```python
from build123d import *

# Parameters (mm, degrees)
F1_DEPTH = 5


# Not quite as in the source:
# - a feature of the source that left no trace in its solid (it failed there, or was rolled back) is left out


with BuildPart() as f1:
    # F0 (on Front) → F1 (new body)
    with BuildSketch(Plane.XZ):
        Polygon((32.530919835, 39.797769749), (-17.469080165, 39.797769749), (-17.469080165, 33.1753157079), (-7.3289242573, 33.1753157079), (22.6710757427, 33.1753157079), (32.530919835, 33.1753157079), align=None)
        with BuildLine():
            Line((22.6710757427, 33.1753157079), (-7.3289242573, 33.1753157079))
            ThreePointArc((-7.3289242573, 33.1753157079), (-3.5071800034, 30.8135939836), (0.6755496306, 29.1740112764))
            Line((0.6755496306, 29.1740112764), (7.6710757427, 29.1740112764))
            Line((7.6710757427, 29.1740112764), (14.6666018548, 29.1740112764))
            ThreePointArc((14.6666018548, 29.1740112764), (18.8493314888, 30.8135939836), (22.6710757427, 33.1753157079))
        make_face()
        with BuildLine():
            Line((7.6710757427, 29.1740112764), (0.6755496306, 29.1740112764))
            ThreePointArc((0.6755496306, 29.1740112764), (0.5215760436, 24.0947560366), (5.6017371537, 24.215191712))
            ThreePointArc((5.6017371537, 24.215191712), (6.355285365, 26.8119146366), (7.6710757427, 29.1740112764))
        make_face()
        with BuildLine():
            ThreePointArc((9.7404143316, 24.215191712), (15.0089010531, 23.907669722), (14.6666018548, 29.1740112764))
            Line((14.6666018548, 29.1740112764), (7.6710757427, 29.1740112764))
            ThreePointArc((7.6710757427, 29.1740112764), (8.9868661204, 26.8119146366), (9.7404143316, 24.215191712))
        make_face()
        with BuildLine():
            ThreePointArc((9.7404143316, 24.215191712), (8.9868661204, 26.8119146366), (7.6710757427, 29.1740112764))
            ThreePointArc((7.6710757427, 29.1740112764), (6.355285365, 26.8119146366), (5.6017371537, 24.215191712))
            ThreePointArc((5.6017371537, 24.215191712), (5.7343151874, 19.5038742549), (7.6710757427, 15.20700939))
            ThreePointArc((7.6710757427, 15.20700939), (9.607836298, 19.5038742549), (9.7404143316, 24.215191712))
        make_face()
    extrude(amount=F1_DEPTH)


solid = f1.part
```
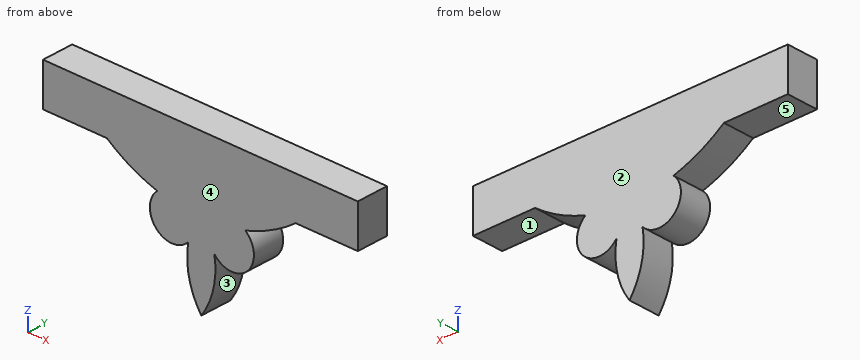
Model file for the job. Use its own axes, mm. Face numbers are marked on the shaded views. A direction names the side the tool comes from. Coordinates: 2 decimals unless noted, no trailing zeros. Order: outer loops, then holes, each group sorted by start corner. A loop starts at its lowest first (then second) coordinate and runs counter-clockwise, first axis right, second up. Notation, with made-up numbers: (-9, 52.5) - (33, 52.5) arc R24 ccw to (33, 81.5) - close; hole circle Ø5 at (-32.75, -15.5). An arc over 180 degrees is marked (long way). Return JSON: item names as keys, results as strings. Group by question number.
1) Saw through at A-A, the plane y = -1.3. Write the cut outline in (x, z).
2) Saw through at B-B, the plane x = 15.5. Write the cut outline in (y, z).
3) Probe line 1 (X direction, y = -4.4, z = 23.5); line 2 (Z direction, x = -10, y = -3.4); line 3 (X direction, y = -4.55, z = 24.75). List the from-to ranges inside material, lowest first. Write a range as from..to.
4) Saw through at D-D, the plane z = 31.5. Write the cut outline in (x, y), plus the area to 3 significant figures.
5) Tool access for the marked faces 1 and 2: list every direction of +Z, -Z, +X, -X, +Y, -Y with a clear straight run to the whole face (end or side of a thin tool).
6) Saw through at C-C, the plane x = 27.5. Write the cut outline in (y, z).
7) Flat gauge pins, fed straight in: P1, Ø2.5, axis at x = -15, y = -3, coming from the -Z side; P2, Ø3, axis at x = 15.5, y = -1, coming from the -Z side; P3, Ø1, axis at x = 20.5, y = -4, coming from the -Z side. Where does each tip first touch, or does it go through?
8) Mould opens along Z. For the marked faces 3, 4 and 5 say: released by +Z, released by -Z, zero draft, split by the parting line, or undercut.
Values found:
{
 "1": {"outline": "(-17.47, 33.18) - (-7.33, 33.18) arc R25 ccw to (0.68, 29.17) arc R3.5 ccw (long way) to (5.6, 24.22) arc R12 ccw to (7.67, 15.21) arc R12 ccw to (9.74, 24.22) arc R3.52 ccw (long way) to (14.67, 29.17) arc R25 ccw to (22.67, 33.18) - (32.53, 33.18) - (32.53, 39.8) - (-17.47, 39.8) - close"},
 "2": {"outline": "(-5, 24.53) - (0, 24.53) - (0, 28.25) - (-5, 28.25) - close; (-5, 29.43) - (0, 29.43) - (0, 39.8) - (-5, 39.8) - close"},
 "3": {"line 1": "x = 1.31..4.7, 5.5..9.84, 10.5..14.52", "line 2": "z = 33.18..39.8", "line 3": "x = 0.01..15.63"},
 "4": {"outline": "(-4.79, -5) - (20.13, -5) - (20.13, 0) - (-4.79, 0) - close", "area": "125 mm²"},
 "5": {"face 1": "-Z, +X, +Y, -Y", "face 2": "+Z, -Z, +X, -X, +Y"},
 "6": {"outline": "(-5, 33.18) - (0, 33.18) - (0, 39.8) - (-5, 39.8) - close"},
 "7": {"P1": "stops at z = 33.18", "P2": "stops at z = 23.2", "P3": "stops at z = 31.43"},
 "8": {"face 3": "undercut", "face 4": "zero draft", "face 5": "released by -Z"}
}
